from build123d import *

# Parameters (mm, degrees)
BOSS_EXTRUDE1_DEPTH     = 4.7625
SKETCH2_R               = 3.96875
SKETCH2_R_2             = 15.875
CUT_EXTRUDE1_DEPTH      = 1
CUT_EXTRUDE1_DEPTH_BACK = 5.7625
F_10_CLEARANCE_HOLE2_D  = 4.9784
CUT_EXTRUDE3_DEPTH      = 5.7625
CUT_EXTRUDE4_DEPTH      = 5.7625
FILLET1_R               = 4
LPATTERN1_COUNT         = 4
LPATTERN1_PITCH         = 90
FILLET1_OF_LPATTERN1_R  = 4
CUT_EXTRUDE5_DEPTH      = 5.7625
FILLET2_R               = 4
LPATTERN2_COUNT         = 3
LPATTERN2_PITCH         = 90
FILLET2_OF_LPATTERN2_R  = 4
SKETCH13_R              = 13.96875
SKETCH13_R_2            = 3.96875
BOSS_EXTRUDE2_DEPTH     = 4.7625
FILLET3_R               = 20


with BuildPart() as part:
    # Sketch1 → Boss-Extrude1 (new body)
    with BuildSketch(Plane.XY):
        with BuildLine():
            Line((-225, 35), (225, 35))
            ThreePointArc((225, 35), (260, 0), (225, -35))
            Line((225, -35), (-225, -35))
            ThreePointArc((-225, -35), (-260, 0), (-225, 35))
        make_face()
    extrude(amount=BOSS_EXTRUDE1_DEPTH)

    # Sketch2 → Cut-Extrude1 (cut, two sides)
    with BuildSketch(Plane(origin=(0, 0, 0), x_dir=(-1, 0, 0), z_dir=(0, 0, -1))) as cut_extrude1_sk:
        with Locations((-145, 18.1)):
            Circle(SKETCH2_R)
        with Locations((135, 18.1)):
            Circle(SKETCH2_R)
        with Locations((-225, 0)):
            Circle(SKETCH2_R_2)
        with Locations((225, 0)):
            Circle(SKETCH2_R_2)
    extrude(amount=CUT_EXTRUDE1_DEPTH, mode=Mode.SUBTRACT)
    extrude(cut_extrude1_sk.sketch, amount=-CUT_EXTRUDE1_DEPTH_BACK, mode=Mode.SUBTRACT)

    # #10 Clearance Hole2 (through all)
    with Locations(Plane.XY.offset(4.7625)):
        with Locations((-180, -25), (-90, -25), (0, -25), (90, -25)):
            Hole(F_10_CLEARANCE_HOLE2_D / 2)

    # Sketch16 → Cut-Extrude3 (cut, through all)
    with BuildSketch(Plane.XY.offset(4.7625)):
        with BuildLine():
            Line((-207.139708849, 30.1), (207.139708849, 30.1))
            ThreePointArc((207.139708849, 30.1), (215.739870411, 33.752777663), (225, 35))
            Line((225, 35), (-225, 35))
            ThreePointArc((-225, 35), (-215.739870411, 33.752777663), (-207.139708849, 30.1))
        make_face()
    extrude(amount=-CUT_EXTRUDE3_DEPTH, mode=Mode.SUBTRACT)

    # Sketch17 → Cut-Extrude4 (cut, through all)
    with BuildSketch(Plane.XY.offset(4.7625)):
        Polygon((-106.063328248, -20), (-135, 7.714901167), (-163.936671752, -20), align=None)
    cut_extrude4 = extrude(amount=-CUT_EXTRUDE4_DEPTH, mode=Mode.SUBTRACT)

    # Fillet1
    fillet1_edges = [part.edges().sort_by_distance(p)[0] for p in [
        (-163.936671752, -20, 2.38125),
        (-135, 7.714901167, 2.38125),
        (-106.063328248, -20, 2.38125),
    ]]
    fillet(fillet1_edges, radius=FILLET1_R)

    # LPattern1: Cut-Extrude4 ×4
    with Locations(*[(i * LPATTERN1_PITCH, 0, 0) for i in range(1, LPATTERN1_COUNT)]):
        add(cut_extrude4, mode=Mode.SUBTRACT)

    # Fillet1 of LPattern1
    fillet1_of_lpattern1_edges = [part.edges().sort_by_distance(p)[0] for p in [
        (-73.936671752, -20, 2.38125),
        (-45, 7.714901167, 2.38125),
        (-16.063328248, -20, 2.38125),
        (16.063328248, -20, 2.38125),
        (45, 7.714901167, 2.38125),
        (73.936671752, -20, 2.38125),
        (106.063328248, -20, 2.38125),
        (135, 7.714901167, 2.38125),
        (163.936671752, -20, 2.38125),
    ]]
    fillet(fillet1_of_lpattern1_edges, radius=FILLET1_OF_LPATTERN1_R)

    # Sketch18 → Cut-Extrude5 (cut, through all)
    with BuildSketch(Plane.XY.offset(4.7625)):
        Polygon((-90, -14.614901167), (-58.975161195, 15.1), (-121.024838805, 15.1), align=None)
    cut_extrude5 = extrude(amount=-CUT_EXTRUDE5_DEPTH, mode=Mode.SUBTRACT)

    # Fillet2
    fillet2_edges = [part.edges().sort_by_distance(p)[0] for p in [
        (-121.024838805, 15.1, 2.38125),
        (-58.975161195, 15.1, 2.38125),
        (-90, -14.614901167, 2.38125),
    ]]
    fillet(fillet2_edges, radius=FILLET2_R)

    # LPattern2: Cut-Extrude5 ×3
    with Locations(*[(i * LPATTERN2_PITCH, 0, 0) for i in range(1, LPATTERN2_COUNT)]):
        add(cut_extrude5, mode=Mode.SUBTRACT)

    # Fillet2 of LPattern2
    fillet2_of_lpattern2_edges = [part.edges().sort_by_distance(p)[0] for p in [
        (-31.024838805, 15.1, 2.38125),
        (31.024838805, 15.1, 2.38125),
        (0, -14.614901167, 2.38125),
        (58.975161195, 15.1, 2.38125),
        (121.024838805, 15.1, 2.38125),
        (90, -14.614901167, 2.38125),
    ]]
    fillet(fillet2_of_lpattern2_edges, radius=FILLET2_OF_LPATTERN2_R)

    # Sketch13 → Boss-Extrude2 (add)
    with BuildSketch(Plane.XY.offset(4.7625)):
        with Locations((-135, 18.1)):
            Circle(SKETCH13_R)
        with Locations((-135, 18.1)):
            Circle(SKETCH13_R_2, mode=Mode.SUBTRACT)
        with Locations((145, 18.1)):
            Circle(SKETCH13_R)
        with Locations((145, 18.1)):
            Circle(SKETCH13_R_2, mode=Mode.SUBTRACT)
    extrude(amount=-BOSS_EXTRUDE2_DEPTH)

    # Fillet3
    fillet3_edges = [part.edges().sort_by_distance(p)[0] for p in [
        (-207.139708849, 30.1, 2.38125),
        (207.139708849, 30.1, 2.38125),
    ]]
    fillet(fillet3_edges, radius=FILLET3_R)


solid = part.part
Input: part model. Units: mm. Frame: model coordinates. A direction names the side the tool comes from. Round coordinates to 2 decimals unless told otherwise and drop trailing zeros. Order: outer loops, then holes, each group sorted by start corner. A loop starts at its lowest first (then second) coordinate and runs counter-clockwise, first axis right, second up.
1. Pin query (flat end, axial travel): P1, Ø1.5, axis at y = 27.5, z = 0.5, coming from the -X side; P2, Ø2.5, axis at x = 0, z = 2.5, coming from the +Y side; P3, Ø1, axis at x = -152, y = -22, coming from the -Z side. Return the tip coordinate at first contact, or that it passes through.
The answers:
P1: stops at x = -247.57
P2: stops at y = 30.1
P3: stops at z = 0
2. Set-up query: faces 1 (the face through (-122.34, -4.41, 2.41)), 2 (the face through (4, -15, 4.762)). Return all of +Z, -Z, +X, -X, +Y, -Y with unobstructed straight access to the full face (end or side cutting, diameter ignored); none if empty.
The answers:
face 1: +Z, -Z
face 2: +Z, +X, -X, +Y, -Y
3. Cut plane B-B, the plane x = -188. Output: boundary loops of the cut face in (y, z), then the cut area to 3 significant figures.
The answers:
outline: (-35, 0) - (30.1, 0) - (30.1, 4.76) - (-35, 4.76) - close
area: 310 mm2
4. Cut plane A-A, the plane z = 2.9. State how many separate pieces and enclosed holes the cut face has, then the cut area to 3 significant figures.
The answers:
separate pieces: 1
enclosed holes: 15
area: 25,900 mm2
5. Mould query, pull axis X, two halves, no side actions, for faces 3 (the face through (4, -15, 0)), 4 (the face through (-32.61, -4.15, 2.41)). Classes: released by +X, released by -X, zero draft, split by the parting line, or undercut.
The answers:
face 3: zero draft
face 4: undercut
6. Material intervals for line 1 (Y direction, x = 0, z = 3.35); line 2 (Y direction, x = -180, z = 1.75); line 3 (X direction, y = -19.5, z = 3.45), sorted ascending.
The answers:
line 1: y = -35 to -27.49, -22.51 to -13.08, 15.1 to 30.1
line 2: y = -35 to -27.49, -22.51 to 30.1
line 3: x = -254.06 to -155.91, -114.09 to -65.91, -24.09 to 24.09, 65.91 to 114.09, 155.91 to 254.06
